Part print with two shaded views. Sizes in mm from the minimum x, y, z corner. Give positions to 0.01 mm unless a question says otherwise; leave off trailing zeros. Loops run counter-clockwise (first coordinate to the right, second up) from the corner with the lowest first, then second, coordinate; pieces in that order, holes last. Notation, with made-up numbers: M 4,75.25 L 30,75.25 A22 ccw 30,86.25 Z; hole C 27.25,-29.5 d3. An arc over 180 degrees is marked long. Answer in a Markdown table with one row per item.
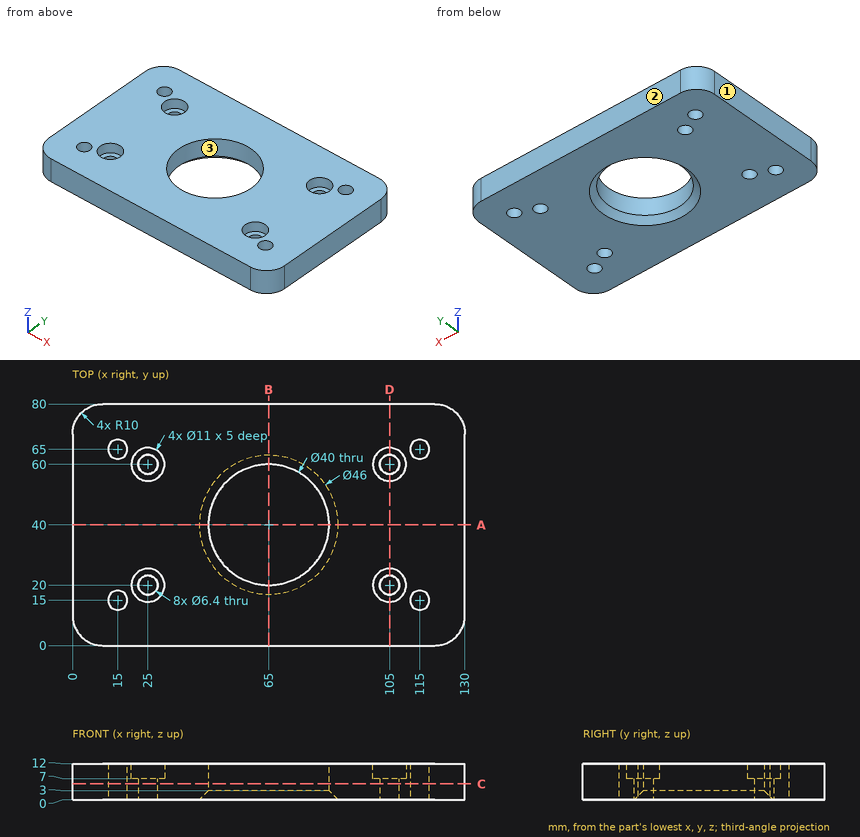
Q1. Saw through at C-C (z = 5.25). Give the number of separate pieces and of enclosed holes in the cut face, and give its area (3 significant figures).
Reported:
| item | result |
|---|---|
| separate pieces | 1 |
| enclosed holes | 9 |
| area | 8,800 mm² |
Q2. Mould opens along Y. For the marked faces 1, 2 and 3 say: released by +Y, released by -Y, zero draft, split by the parting line, or undercut.
Reported:
| item | result |
|---|---|
| face 1 | zero draft |
| face 2 | released by +Y |
| face 3 | undercut |
Q3. Drop a flat-ended pin along its axis: pin 1 (5.5 mm diameter, centred on x = 103, y = 60.5, fed in from +Z). Give the stop position or say it passes through.
Reported:
| item | result |
|---|---|
| pin 1 | z = 7 |
Q4. Saw through at B-B (x = 65). Give the cut face in (y, z).
Reported:
| item | result |
|---|---|
| outline | M 0,0 L 17,0 L 20,3 L 20,12 L 0,12 Z; M 60,3 L 63,0 L 80,0 L 80,12 L 60,12 Z |
Q5. Saw through at D-D (x = 105). Give the cut face in (y, z), and give its area (3 significant figures).
Reported:
| item | result |
|---|---|
| outline | M 0,0 L 16.8,0 L 16.8,7 L 14.5,7 L 14.5,12 L 0,12 Z; M 23.2,0 L 56.8,0 L 56.8,7 L 54.5,7 L 54.5,12 L 25.5,12 L 25.5,7 L 23.2,7 Z; M 63.2,0 L 80,0 L 80,12 L 65.5,12 L 65.5,7 L 63.2,7 Z |
| area | 760 mm² |
Q6. Saw through at A-A (y = 40). Give the cut face in (x, z), and give its area (3 significant figures).
Reported:
| item | result |
|---|---|
| outline | M 0,0 L 42,0 L 45,3 L 45,12 L 0,12 Z; M 85,3 L 88,0 L 130,0 L 130,12 L 85,12 Z |
| area | 1,070 mm² |
Q7. Probe probe 1 along Y at (x, z) = (15, 5.5); probe 2 along Y at (x, z) = (25, 4.75); probe 3 along Y at (x, z) = (65, 9). List the from-to ranges inside material, lowest first.
Reported:
| item | result |
|---|---|
| probe 1 | 0 to 11.8, 18.2 to 61.8, 68.2 to 80 |
| probe 2 | 0 to 16.8, 23.2 to 56.8, 63.2 to 80 |
| probe 3 | 0 to 20, 60 to 80 |
